Input: part model. Units: mm. Frame: model coordinates. Face numbers are marked on the shaded views. Round coordinates to 2 decimals unless told otherwise and drop trailing zeros. Loops run counter-clockwise (first coordinate to the right, second up) from the corner with the lowest first, then second, coordinate; pieces in that order, holes last. Notation, with made-up numbers: (-28.5, -32.75) - (17.5, -32.75) arc R28 ccw to (17.5, 6.25) - close; hole circle Ø8 at (-21.75, 76.5). An arc over 180 degrees is marked (long way). One line per question, with ' | ' between items. Start each with the question number.
from build123d import *
from build123d.topology import SkipClean

# Parameters (mm, degrees)
SKETCH3_W          = 1
SKETCH3_H          = 10
CIRPATTERN1_COUNT  = 6
SKETCH5_R          = 11
SKETCH5_R_2        = 10
CUT_EXTRUDE1_DEPTH = 4


with BuildPart() as part:
    # Sketch3 → Revolve3 (revolve)
    with BuildSketch(Plane.XY, mode=Mode.PRIVATE) as revolve3_sk:
        with Locations((10.5, 0)):
            Rectangle(SKETCH3_W, SKETCH3_H)
    revolve(revolve3_sk.sketch.rotate(Axis((0, 0, 0), (0, 1, 0)), 90), axis=Axis((0, 0, 0), (0, 1, 0)))

    # Sketch4 → Cut-Revolve1 (revolve, cut)
    with SkipClean():  # the faces are left unmerged after this step: merging them gives an invalid solid
        with BuildSketch(Plane.XY, mode=Mode.PRIVATE) as cut_revolve1_sk:
            with BuildLine():
                ThreePointArc((10.5, 2.2), (8.3, 0), (10.5, -2.2))
                Line((10.5, -2.2), (10.5, 2.2))
            make_face()
            with BuildLine():
                Line((10.5, 2.2), (10.5, -2.2))
                ThreePointArc((10.5, -2.2), (12.055634919, -1.555634919), (12.7, 0))
                ThreePointArc((12.7, 0), (12.055634919, 1.555634919), (10.5, 2.2))
            make_face()
        cut_revolve1 = revolve(cut_revolve1_sk.sketch.rotate(Axis((10.5, -2.2, 0), (0, 1, 0)), 264.14281938), axis=Axis((10.5, -2.2, 0), (0, 1, 0)), mode=Mode.SUBTRACT)
    add(part.part.scale(1), mode=Mode.REPLACE)  # the faces are merged on a copy

    # CirPattern1: Cut-Revolve1 ×6 about axis
    cirpattern1_axis = Axis((0, 0, 0), (0, 1, 0))
    for i in range(1, CIRPATTERN1_COUNT):
        add(cut_revolve1.rotate(cirpattern1_axis, i * 360 / CIRPATTERN1_COUNT), mode=Mode.SUBTRACT)

    # Sketch5 → Cut-Extrude1 (cut)
    with BuildSketch(Plane(origin=(0, 5, 0), x_dir=(1, 0, 0), z_dir=(0, 1, 0))):
        with Locations(Location((0, 0, 0), (0, 0, 90))):
            Circle(SKETCH5_R)
        with Locations(Location((0, 0, 0), (0, 0, 90))):
            Circle(SKETCH5_R_2, mode=Mode.SUBTRACT)
    extrude(amount=-CUT_EXTRUDE1_DEPTH, mode=Mode.SUBTRACT)


solid = part.part
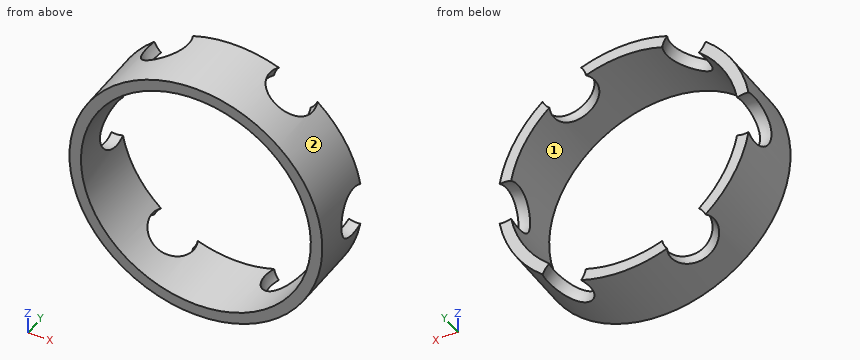
(1) Pin query (flat end, axial travel): P1, Ø1.5, axis at x = 3, y = -3.5, coming from the +Z side; P2, Ø1.5, axis at x = 4.5, y = -1.5, coming from the +Z side; P3, Ø1.5, axis at y = -1, z = -8, coming from the -X side. Return the tip coordinate at first contact, or that it passes through.
(2) Pull-direction query (X, two-part tool) for the marked faces 1 and 2; classes: released by +X, released by -X, zero draft, split by the parting line, or undercut.
(3) Section B-B, the plane z = 4.25. Output: boundary loops of the cut face in (x, y), plus the area to 3 significant figures.
(4) Section C-C, the plane y = -3.5. Output: boundary loops of the cut face in (x, z), plus the area to 3 significant figures.
(5) Section A-A, the plane x = 0. Output: boundary loops of the cut face in (y, z), plus the area to 3 significant figures.
(6) Line query: line 1 along X through (y, z) = (-2.75, 0); line 2 along X through (y, z) = (-4.25, 8.5); line 3 along Z through (x, y) = (-7, 0.75). Output: solid intervals per line, ascending. Write a range as from..to.
Derived:
1) P1: stops at z = 10.77 | P2: stops at z = 10.34 | P3: stops at x = -8.27
2) face 1: undercut | face 2: split by the parting line
3) outline: (-10.15, -5) - (-9.05, -5) - (-9.05, 1) - (-10.15, 1) - close; (9.05, -5) - (10.15, -5) - (10.15, 1) - (9.05, 1) - close | area: 13.1 mm²
4) outline: circle Ø22 at (0, 0); hole circle Ø20 at (0, 0) | area: 66.0 mm²
5) outline: (-5, -11) - (1, -11) - (1, -10) - (-5, -10) - close; (-5, 10) - (1, 10) - (1, 11) - (-5, 11) - close | area: 12.0 mm²
6) line 1: x = -11..-10, 10..11 | line 2: x = -6.98..-5.27, 5.27..6.98 | line 3: z = -7.99..-7.14, 7.14..7.99
